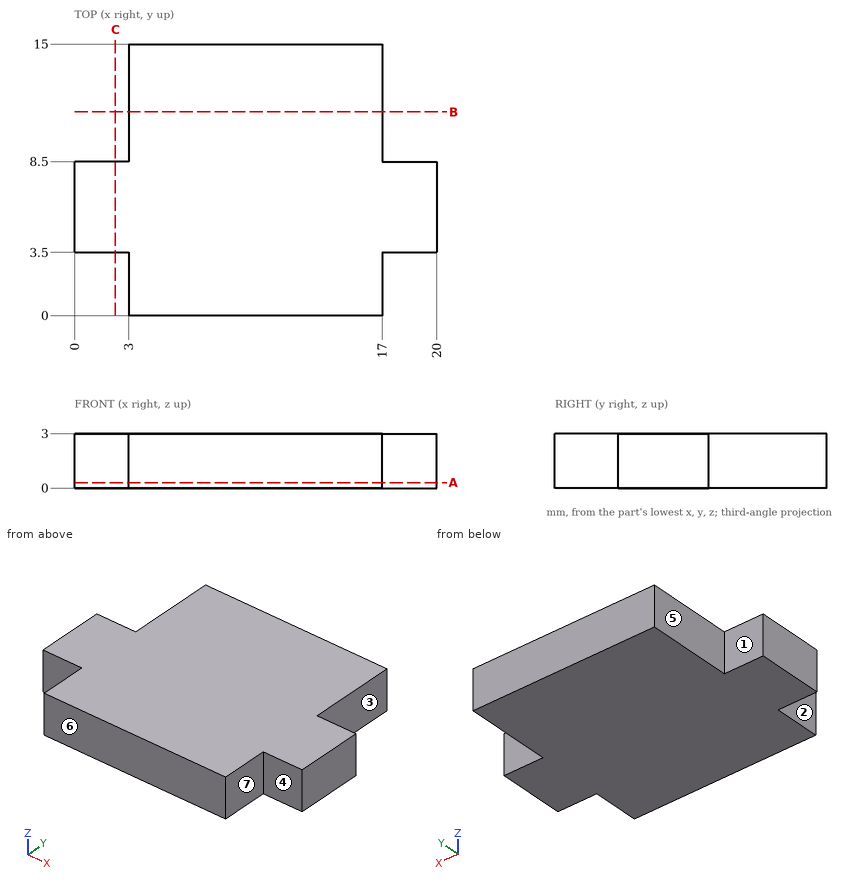
Study the drawing (mm; zero at the part's minimum x, y, z) and answer. A direction names the side the tool comes from. Round coordinates to 2 decimals unless told otherwise and drop trailing zeros. Write each loop counter-clockwise with the first axis right and the second up, starting at its lowest first coordinate (ties: lowest second). Pieces come first, ordered by that corner, then holes. Notation, with made-up numbers: (49, 75.5) - (97, 75.5) arc R18 cw to (97, 102.5) - close; hole circle Ø10 at (-5, 37.5). An arc over 180 degrees is marked (long way). Return JSON: item names as keys, results as strings. Group by question number.
Q1. Each of these flat-tipped pins is pushed along its axis until it touches: pin 1 Ø1.5 at (x, z) = (19, 1.5) entering from +Y; pin 2 Ø0.9 at (y, z) = (1, 1) entering from +X; pin 3 Ø0.9 at (y, z) = (12.5, 1.5) entering from -X. Where does it stop, or does it pass through?
Q2. The part is cut by section A-A on z = 0.3. Write down the section's boundary in (x, y), then the cut area to 3 significant figures.
Q3. The part is cut by section C-C on x = 2.25. Write down the section's boundary in (y, z), then the cut area to 3 significant figures.
Q4. The part is cut by section B-B on y = 11.25. Write down the section's boundary in (x, z).
Q5. The mould has two halves that part along X. Classify the marked faces 5, 6 and 7: released by +X, released by -X, zero draft, split by the parting line, or undercut.
Q6. For the marked faces 1, 2, 3 and 4, determine the directions among +Z, -Z, +X, -X, +Y, -Y from which every point of the face is accessible in a straight line to the end or side of a thin tool.
Q7. Find the intervals of material crossed by L1, parallel to X at y = 3, z = 1.9; L2, parallel to Y at x = 2.5, z = 2.45, in increasing order.
Solved:
{
 "1": {"pin 1": "y = 8.5", "pin 2": "x = 17", "pin 3": "x = 3"},
 "2": {"outline": "(0, 3.5) - (3, 3.5) - (3, 0) - (17, 0) - (17, 3.5) - (20, 3.5) - (20, 8.5) - (17, 8.5) - (17, 15) - (3, 15) - (3, 8.5) - (0, 8.5) - close", "area": "240 mm²"},
 "3": {"outline": "(3.5, 0) - (8.5, 0) - (8.5, 3) - (3.5, 3) - close", "area": "15.0 mm²"},
 "4": {"outline": "(3, 0) - (17, 0) - (17, 3) - (3, 3) - close"},
 "5": {"face 5": "released by -X", "face 6": "zero draft", "face 7": "released by +X"},
 "6": {"face 1": "+Z, -Z, -X, +Y", "face 2": "+Z, -Z, -X, -Y", "face 3": "+Z, -Z, +X, +Y", "face 4": "+Z, -Z, +X, -Y"},
 "7": {"L1": "3 to 17", "L2": "3.5 to 8.5"}
}
